Input: part model. Units: mm. Frame: model coordinates. A direction names the side the tool comes from. Round coordinates to 2 decimals unless told otherwise and drop trailing zeros. Loops run counter-clockwise (first coordinate to the right, second up) from the corner with the lowest first, then second, coordinate; pieces in that order, holes last. Notation, with made-up numbers: M 49,68.25 L 108,68.25 A24 cw 108,87.25 Z; hole C 30,26.5 d9. An arc over 180 degrees is marked long. Put each result on its own line as item: value. Start each with the question number.
1) Section A-A on z = -8.5. Output: boundary loops of the cut face in (x, y), plus the area to 3 significant figures.
2) Reachability of faces 1 (the face through (94.6, 1, 22.3)), 2 (the face through (-5.5, 1, 15)), 3 (the face through (1, 1, -24.345)) from +Z, -Z, +X, -X, +Y, -Y: full face, straight path, thin tool, end or side. Return the list, or none.
3) Line query: probe 1 along Z at (x, y) = (0, 2.55); probe 2 along X at (y, z) = (2.8, 12.5); probe 3 along Z at (x, y) = (59.5, 2.55). Output: solid intervals per line, ascending.
4) Draft query along X for faces 4 (the face through (95, 1, 5)), 5 (the face through (-90.4, 1, 22.3)), 6 (the face through (0, 3, -18)), 7 (the face through (-95, 1, 5)). Return one class per face: +X half, -X half, draft (parallel to the pull), parting line (faces both ways), or undercut.
5) Pin query (flat end, axial travel): pin 1 (1.3 mm diameter, centred on x = -93, z = 21, fed in from -Y); pin 2 (5 mm diameter, centred on x = 16.5, z = -3.5, fed in from +Y); pin 3 (2 mm diameter, centred on x = -92.5, z = 21.85, fed in from +Y). Return the tip coordinate at first contact, or that it passes through.
6) Section B-B on x = -31.5. Output: boundary loops of the cut face in (y, z).
7) Section C-C on y = 1.05. State how many separate pieces and enclosed holes the cut face has, plus the area to 3 significant figures.
from build123d import *

# Parameters (mm, degrees)
EXTRUDE_2_DEPTH          = 3
HOLE_WIZARD_6_AT_2_COUNT = 2
HOLE_WIZARD_6_AT_2_PITCH = 102.259107828
HOLE_WIZARD_6_AT_3_COUNT = 2
HOLE_WIZARD_6_AT_3_PITCH = 185
SKETCH_15_W              = 11
SKETCH_15_H              = 8
CUT_EXTRUDE_1_DEPTH      = 99.115732766
SHELL_START              = 2
SHELL_3_OUTLINE_W        = 15
SHELL_3_OUTLINE_H        = 12
SHELL_3_DEPTH            = 1


# Read off the part's stored shape, not the designer's step: 抽壳3
with BuildPart() as part:
    # 草图1 → 凸台-拉伸2 (new body)
    with BuildSketch(Plane(origin=(0, 0, 0), x_dir=(1, 0, 0), z_dir=(0, 1, 0))):
        with BuildLine():
            Line((85, 24.345368999), (-85, 24.345368999))
            add(Edge.make_bspline(
                [(-85, 24.345368999), (-95, 24.345368999), (-95, 13.969349259)],
                knots=[0, 0, 0, 1.570796327, 1.570796327, 1.570796327], degree=2, weights=[1, 0.707106781, 1]))
            Line((-95, 13.969349259), (-95, -24.345368999))
            Line((-95, -24.345368999), (95, -24.345368999))
            Line((95, -24.345368999), (95, 13.969349259))
            add(Edge.make_bspline(
                [(95, 13.969349259), (95, 24.345368999), (85, 24.345368999)],
                knots=[1.570796327, 1.570796327, 1.570796327, 3.141592654, 3.141592654, 3.141592654], degree=2, weights=[1, 0.707106781, 1]))
        make_face()
    extrude(amount=EXTRUDE_2_DEPTH)

    # 草图14 → 大小六角凹头盖螺钉柱孔6 (revolve, cut)
    with BuildSketch(Plane(origin=(92.5, 0, 21.845368999), x_dir=(0, 0, -1), z_dir=(1, 0, 0))):
        Polygon((0, 0), (0, 3), (1.2, 3), (1.2, 2), (2.15, 2), (2.15, 0.024142219), (2.175, 0), align=None)
    hole_wizard_6 = revolve(axis=Axis((92.5, -6.35, 21.845368999), (0, 1, 0)), mode=Mode.SUBTRACT)

    # 大小六角凹头盖螺钉柱孔6 at 2: 大小六角凹头盖螺钉柱孔6 ×2
    with Locations(*[Vector(-0.9045649034602262, 0, -0.42633594198471203) * (i * HOLE_WIZARD_6_AT_2_PITCH) for i in range(1, HOLE_WIZARD_6_AT_2_COUNT)]):
        add(hole_wizard_6, mode=Mode.SUBTRACT)

    # 大小六角凹头盖螺钉柱孔6 at 3: 大小六角凹头盖螺钉柱孔6 ×2
    with Locations(*[(-i * HOLE_WIZARD_6_AT_3_PITCH, 0, 0) for i in range(1, HOLE_WIZARD_6_AT_3_COUNT)]):
        add(hole_wizard_6, mode=Mode.SUBTRACT)

    # 草图15 → 切除-拉伸1 (cut, through all)
    with BuildSketch(Plane.XZ):
        with Locations((0, 15.345368999)):
            Rectangle(SKETCH_15_W, SKETCH_15_H)
    extrude(amount=-CUT_EXTRUDE_1_DEPTH, mode=Mode.SUBTRACT)

    # 抽壳3 outline → 抽壳3 (cut)
    with BuildSketch(Plane(origin=(0, 0, 0), x_dir=(1, 0, 0), z_dir=(0, 1, 0)).offset(SHELL_START)):
        with BuildLine():
            Line((93, -17.725599588), (93.000000196, 13.969349259))
            add(Edge.make_bspline(
                [(93.000000196, 13.969349259), (93.000000196, 14.990185456), (92.871215367, 16.011021653), (92.613645709, 17.01184643), (92.230602513, 17.972648367), (91.728708361, 18.874166906), (91.117678233, 19.698643208), (90.409881727, 20.430484444), (89.619725312, 21.056754945), (88.762932516, 21.567410906), (87.855861705, 21.955201909), (86.915108734, 22.215310689), (85.957556964, 22.345368999), (85, 22.345368999)],
                knots=[1.570796327, 1.570796327, 1.570796327, 1.570796327, 1.570796327, 1.570796327, 1.570796327, 1.570796327, 1.570796327, 1.570796327, 1.570796327, 1.570796327, 1.570796327, 1.570796327, 3.141592654, 3.141592654, 3.141592654, 3.141592654, 3.141592654, 3.141592654, 3.141592654, 3.141592654, 3.141592654, 3.141592654, 3.141592654, 3.141592654, 3.141592654, 3.141592654], degree=13))
            Line((85, 22.345368999), (4.107268939, 22.345368999))
            ThreePointArc((4.107268939, 22.345368999), (0, 17.601364064), (-4.107268939, 22.345368999))
            Line((-4.107268939, 22.345368999), (-85, 22.345368999))
            add(Edge.make_bspline(
                [(-85, 22.345368999), (-85.957556964, 22.345368999), (-86.915108734, 22.215310689), (-87.855861705, 21.955201909), (-88.762932516, 21.567410906), (-89.619725312, 21.056754945), (-90.409881727, 20.430484444), (-91.117678233, 19.698643208), (-91.728708361, 18.874166906), (-92.230602513, 17.972648367), (-92.613645709, 17.01184643), (-92.871215367, 16.011021653), (-93.000000196, 14.990185456), (-93.000000196, 13.969349259)],
                knots=[0, 0, 0, 0, 0, 0, 0, 0, 0, 0, 0, 0, 0, 0, 1.570796327, 1.570796327, 1.570796327, 1.570796327, 1.570796327, 1.570796327, 1.570796327, 1.570796327, 1.570796327, 1.570796327, 1.570796327, 1.570796327, 1.570796327, 1.570796327], degree=13))
            Line((-93.000000196, 13.969349259), (-93, -17.725599588))
            ThreePointArc((-93, -17.725599588), (-89.565506858, -18.910875857), (-88.380230589, -22.345368999))
            Line((-88.380230589, -22.345368999), (88.380230589, -22.345368999))
            ThreePointArc((88.380230589, -22.345368999), (89.565506858, -18.910875857), (93, -17.725599588))
        make_face()
        with Locations((0, -15.345368999)):
            Rectangle(SHELL_3_OUTLINE_W, SHELL_3_OUTLINE_H, mode=Mode.SUBTRACT)
    extrude(amount=SHELL_3_DEPTH, mode=Mode.SUBTRACT)


solid = part.part
Geometry results:
1. outline: M -95,0 L 95,0 L 95,3 L 93,3 L 93,2 L -93,2 L -93,3 L -95,3 Z
1. area: 384 mm²
2. face 1: -Y
2. face 2: +Y, -Y
2. face 3: -Z, +X, -X, +Y, -Y
3. probe 1: z = -24.35 to -22.95, -20.55 to -17.6, 9.35 to 11.35, 19.35 to 21.35, 22.35 to 24.35
3. probe 2: x = -95 to -93, -7.5 to -5.5, 5.5 to 7.5, 93 to 95
3. probe 3: z = -24.35 to -22.35, 22.35 to 24.35
4. face 4: +X half
4. face 5: undercut
4. face 6: draft
4. face 7: -X half
5. pin 1: stops at y = 2
5. pin 2: stops at y = 2
5. pin 3: passes through
6. outline: M 0,-24.35 L 3,-24.35 L 3,-22.35 L 2,-22.35 L 2,22.35 L 3,22.35 L 3,24.35 L 0,24.35 Z
7. separate pieces: 1
7. enclosed holes: 4
7. area: 9,080 mm²
